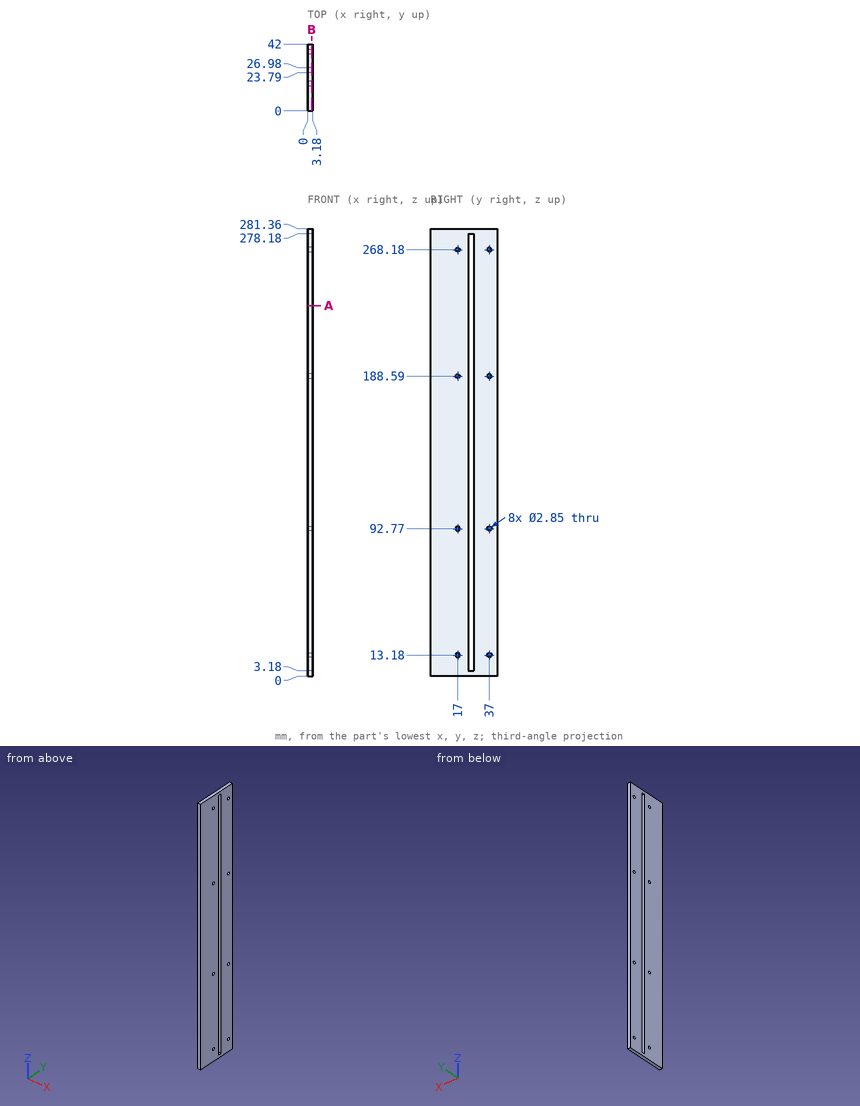
The figure shows three views and two pictorial views of one solid part (mm, origin at its lowest corner). Answer the questions. Coordinates: 2 decimals unless noted, no trailing zeros. Loops run counter-clockwise (first coordinate to the right, second up) from the corner with the lowest first, then second, coordinate; pieces in that order, holes last.
1) Flat-ended cylindrical pins translate along their axes: pin 1 Ø3.5 at (y, z) = (37, 92.77) entering from -X; pin 2 Ø2.5 at (y, z) = (17, 92.77) entering from +X (3 decimals). Find the tip coordinate at first contact, or state that the pin passes through.
2) Find section B-B on x = 2.5. Give the number of separate pieces and of enclosed holes in the cut face, then the cut area to 3 significant figures.
3) Find section A-A on z = 233. Write down the section's boundary in (x, y), then the cut area to 3 significant figures.
4) Find the intervals of material crossed by L1, parallel to Y at x = 0.6, z = 268.18 (3 decimals); L2, parallel to Z at x = 1.3, y = 17 (3 decimals); L3, parallel to Y at x = 1.3, z = 147, in increasing order.
Values:
1. pin 1: stops at x = 0
1. pin 2: passes through
2. separate pieces: 1
2. enclosed holes: 9
2. area: 10,900 mm2
3. outline: (0, 0) - (3.18, 0) - (3.18, 23.79) - (0, 23.79) - close; (0, 26.98) - (3.18, 26.98) - (3.18, 42) - (0, 42) - close
3. area: 123 mm2
4. L1: y = 0 to 15.575, 18.425 to 23.79, 26.98 to 35.575, 38.425 to 42
4. L2: z = 0 to 11.755, 14.605 to 91.345, 94.195 to 187.165, 190.015 to 266.755, 269.605 to 281.36
4. L3: y = 0 to 23.79, 26.98 to 42
